Model file for the job. Use its own axes, mm. Give positions to 0.01 mm unless a question says otherwise; leave off trailing zeros. Loops run counter-clockwise (first coordinate to the right, second up) from the corner with the lowest first, then second, coordinate; pieces in that order, holes last. Notation, with made-up numbers: (29, 48) -> (57, 48) arc R19 ccw to (57, 76) -> close; hole circle Ø6 at (47, 10). An arc over 180 degrees is marked (long way). Use CSV: the item, a comma, the result in double quotes. Start each with the question number.
(1) Drill centre lines: probe 1 along Y at (x, z) = (0, 2.15); probe 2 along Y at (x, z) = (-1.75, 2.65); probe 3 along X at (y, z) = (-5, 2.15). Where is each one in solid material? Low to high.
(2) Cut at A-A on y = 6. Write the cut outline in (x, z).
(3) Cut at C-C on z = 2.2. Write the cut outline in (x, y).
(4) Cut at D-D on y = -6. Write the cut outline in (x, z), then the cut area to 3 significant figures.
(5) Pull direction Y, two halves, no side cores. Call faces 1 (the cylindrical face through (0.14, 24.45, 1.48)), 2 (the flat face through (6.45, 0, 1)), 3 (the cylindrical face through (-0.878, 14.046, 1.479)): pulls with the +Y half, pulls with the -Y half, needs draft (parallel to the pull), parting line crosses it, or undercut.
(6) Flat gauge pin, fed straight in: pin 1 (6.5 mm diameter, centred on x = 0, y = 18, fed in from -Z). Where does the tip first touch, or does it go through?
(7) Cut at B-B on x = 0. Write the cut outline in (y, z), then the cut area to 3 significant figures.
from build123d import *

# Parameters (mm, degrees)
F0_R     = 2.55
F0_R_2   = 3.05
F0_R_3   = 3.55
F0_R_4   = 4.05
F1_DEPTH = 3


with BuildPart() as f1:
    # F0 (on Top) → F1 (new body)
    with BuildSketch(Plane.XY):
        with BuildLine():
            Line((-6.45, 18), (-6.45, -18))
            ThreePointArc((-6.45, -18), (0, -24.45), (6.45, -18))
            Line((6.45, -18), (6.45, 18))
            ThreePointArc((6.45, 18), (0, 24.45), (-6.45, 18))
        make_face()
        with Locations((0, -18)):
            Circle(F0_R, mode=Mode.SUBTRACT)
        with Locations((0, -6)):
            Circle(F0_R_2, mode=Mode.SUBTRACT)
        with Locations((0, 6)):
            Circle(F0_R_3, mode=Mode.SUBTRACT)
        with Locations((0, 18)):
            Circle(F0_R_4, mode=Mode.SUBTRACT)
    extrude(amount=F1_DEPTH)


solid = f1.part
Check result:
1,probe 1,"-24.45 to -20.55, -15.45 to -9.05, -2.95 to 2.45, 9.55 to 13.95, 22.05 to 24.45"
1,probe 2,"-24.21 to -19.85, -16.15 to -8.5, -3.5 to 2.91, 9.09 to 14.35, 21.65 to 24.21"
1,probe 3,"-6.45 to -2.88, 2.88 to 6.45"
2,outline,"(-6.45, 0) -> (-3.55, 0) -> (-3.55, 3) -> (-6.45, 3) -> close; (3.55, 0) -> (6.45, 0) -> (6.45, 3) -> (3.55, 3) -> close"
3,outline,"(-6.45, -18) arc R6.45 ccw to (6.45, -18) -> (6.45, 18) arc R6.45 ccw to (-6.45, 18) -> close; hole circle Ø8.1 at (0, 18); hole circle Ø7.1 at (0, 6); hole circle Ø6.1 at (0, -6); hole circle Ø5.1 at (0, -18)"
4,outline,"(-6.45, 0) -> (-3.05, 0) -> (-3.05, 3) -> (-6.45, 3) -> close; (3.05, 0) -> (6.45, 0) -> (6.45, 3) -> (3.05, 3) -> close"
4,area,"20.4 mm²"
5,face 1,"pulls with the +Y half"
5,face 2,"needs draft"
5,face 3,"undercut"
6,pin 1,"through"
7,outline,"(-24.45, 0) -> (-20.55, 0) -> (-20.55, 3) -> (-24.45, 3) -> close; (-15.45, 0) -> (-9.05, 0) -> (-9.05, 3) -> (-15.45, 3) -> close; (-2.95, 0) -> (2.45, 0) -> (2.45, 3) -> (-2.95, 3) -> close; (9.55, 0) -> (13.95, 0) -> (13.95, 3) -> (9.55, 3) -> close; (22.05, 0) -> (24.45, 0) -> (24.45, 3) -> (22.05, 3) -> close"
7,area,"67.5 mm²"
